from build123d import *

# Parameters (mm, degrees)
F1_DEPTH = 50


# Not quite as in the source:
# - ends of sketch curves that miss each other by under 0.0002 mm in the source are joined


with BuildPart() as f1:
    # F0 (on Front) → F1 (new body, symmetric)
    with BuildSketch(Plane.XZ):
        with BuildLine():
            Line((53.992555, -15.220268), (57.083133, -14.095389))
            ThreePointArc((57.083133, -14.095389), (62.9018568836, -10.252747544), (66.3544503107, -4.1944440905))
            ThreePointArc((66.3544503107, -4.1944440905), (66.1141142416, -2.8747683688), (64.914288, -2.275))
            Line((64.914288, -2.275), (60.670593, -2.275))
            ThreePointArc((60.670593, -2.275), (59.8472095147, -2.5211899521), (59.2941043505, -3.1789471518))
            ThreePointArc((59.2941043505, -3.1789471518), (56.9827494729, -6.2209259886), (53.52425904, -7.8441451998))
            ThreePointArc((53.52425904, -7.8441451998), (52.6431740995, -8.0626756758), (51.7855370008, -8.3602070021))
            ThreePointArc((51.7855370008, -8.3602070021), (39.452831, 0), (51.7855371982, 8.3602074972))
            ThreePointArc((51.7855371982, 8.3602074972), (52.6431743712, 8.0626765952), (53.524259133, 7.844145664))
            ThreePointArc((53.524259133, 7.844145664), (56.9827494729, 6.2209259886), (59.2941043849, 3.1789471667))
            ThreePointArc((59.2941043849, 3.1789471667), (59.8472095147, 2.5211899521), (60.670593, 2.275))
            Line((60.670593, 2.275), (64.914288, 2.275))
            ThreePointArc((64.914288, 2.275), (66.1141145297, 2.8747687527), (66.3544497778, 4.1944449353))
            ThreePointArc((66.3544497778, 4.1944449353), (62.9018565554, 10.2527478944), (57.0831331177, 14.0953893235))
            Line((57.0831331177, 14.0953893235), (53.992555, 15.220268))
            ThreePointArc((53.992555, 15.220268), (52.3736165632, 15.715360306), (50.7118440801, 16.0387645685))
            Line((50.7118440801, 16.0387645685), (40.585713, 17.465))
            Line((40.585713, 17.465), (35.885713, 17.465))
            ThreePointArc((35.885713, 17.465), (35.6735809656, 17.5528679656), (35.585713, 17.765))
            Line((35.585713, 17.765), (35.585713, 18.7))
            ThreePointArc((35.585713, 18.7), (35.4978450344, 18.9121320344), (35.285713, 19))
            Line((35.285713, 19), (18.585713, 19))
            Line((18.585713, 19), (12.836393, 18.04178))
            ThreePointArc((12.836393, 18.04178), (12.656806899, 17.9397743434), (12.585713, 17.745862))
            Line((12.585713, 17.745862), (12.585713, 6.875))
            ThreePointArc((12.585713, 6.875), (12.6735809656, 6.6628679656), (12.885713, 6.575))
            Line((12.885713, 6.575), (18.285713, 6.575))
            ThreePointArc((18.285713, 6.575), (18.4978450344, 6.6628679656), (18.585713, 6.875))
            Line((18.585713, 6.875), (18.585713, 12.7))
            ThreePointArc((18.585713, 12.7), (18.6735809656, 12.9121320344), (18.885713, 13))
            Line((18.885713, 13), (26.285713, 13))
            ThreePointArc((26.285713, 13), (26.4978450344, 12.9121320344), (26.585713, 12.7))
            Line((26.585713, 12.7), (26.585713, 10.3))
            ThreePointArc((26.585713, 10.3), (26.6735809656, 10.0878679656), (26.885713, 10))
            Line((26.885713, 10), (32.285713, 10))
            ThreePointArc((32.285713, 10), (32.4978450344, 9.9121320344), (32.585713, 9.7))
            Line((32.585713, 9.7), (32.585713, -9.7))
            ThreePointArc((32.585713, -9.7), (32.4978450344, -9.9121320344), (32.285713, -10))
            Line((32.285713, -10), (26.885713, -10))
            ThreePointArc((26.885713, -10), (26.6735809656, -10.0878679656), (26.585713, -10.3))
            Line((26.585713, -10.3), (26.585713, -12.7))
            ThreePointArc((26.585713, -12.7), (26.4978450344, -12.9121320344), (26.285713, -13))
            Line((26.285713, -13), (18.885713, -13))
            ThreePointArc((18.885713, -13), (18.6735809656, -12.9121320344), (18.585713, -12.7))
            Line((18.585713, -12.7), (18.585713, -6.875))
            ThreePointArc((18.585713, -6.875), (18.4978450344, -6.6628679656), (18.285713, -6.575))
            Line((18.285713, -6.575), (12.885713, -6.575))
            ThreePointArc((12.885713, -6.575), (12.6735809656, -6.6628679656), (12.585713, -6.875))
            Line((12.585713, -6.875), (12.585713, -17.745862))
            ThreePointArc((12.585713, -17.745862), (12.656806899, -17.9397743434), (12.8363929795, -18.0417801231))
            Line((12.8363929795, -18.0417801231), (18.585713, -19))
            Line((18.585713, -19), (35.285713, -19))
            ThreePointArc((35.285713, -19), (35.4978450344, -18.9121320344), (35.585713, -18.7))
            Line((35.585713, -18.7), (35.585713, -17.765))
            ThreePointArc((35.585713, -17.765), (35.6735809656, -17.5528679656), (35.885713, -17.465))
            Line((35.885713, -17.465), (40.585713, -17.465))
            Line((40.585713, -17.465), (50.711844, -16.038764))
            ThreePointArc((50.711844, -16.038764), (52.3736165632, -15.715360306), (53.992555, -15.220268))
        make_face()
    extrude(amount=F1_DEPTH, both=True)


solid = f1.part
Read the model definition and answer for the solid it produces. Units are mm, in the model's axes. A direction names the side the tool comes from. Round coordinates to 2 decimals unless told otherwise and drop trailing zeros. Write each loop counter-clockwise with the first axis right and the second up, starting at its lowest first coordinate (ties: lowest second). Pieces come first, ordered by that corner, then holes.
Q1. The mould has two halves that part along Z. Classify faces 1 (the face through (38, -1, -17.465)), 2 (the face through (45.72, -0.7, 16.74)), 3 (the face through (32.586, -1, 0)): released by +Z, released by -Z, zero draft, split by the parting line, or undercut.
Values:
face 1: released by -Z
face 2: released by +Z
face 3: undercut
Q2. Flat-ended cylindrical pins translate along their axes: P1, Ø0.5, axis at y = -6.5, z = 18, coming from the +X side; P2, Ø6, axis at y = -17, z = 3.5, coming from the -X side; P3, Ø1.5, axis at x = 45, y = 13.5, coming from the -Z side. Find the tip coordinate at first contact, or state that the pin passes through.
Values:
P1: stops at x = 35.59
P2: stops at x = 32.59
P3: stops at z = -16.95
Q3. Find section B-B on z = 0. Determine the outline of the cut face in (x, y), and give its area (3 significant figures).
Values:
outline: (32.59, -50) - (39.45, -50) - (39.45, 50) - (32.59, 50) - close
area: 687 mm2
Q4. Find section C-C on x = 63.5. Determine the outline of the cut face in (y, z) (3 decimals).
Values:
outline: (-50, -9.574) - (50, -9.574) - (50, -2.275) - (-50, -2.275) - close; (-50, 2.275) - (50, 2.275) - (50, 9.574) - (-50, 9.574) - close
Q5. Straight lines are drawn through the part: line 1 (Z direction, x = 24, y = -21.5); line 2 (X direction, y = -15, z = 0); line 3 (Z direction, x = 61.5, y = 22) (3 decimals). For each, find the intervals that lie inside material, in ascending order.
Values:
line 1: z = -19 to -13, 13 to 19
line 2: x = 32.59 to 39.45
line 3: z = -11.569 to -2.275, 2.275 to 11.569
Q6. Find section A-A on x = 28.5. Determine the outline of the cut face in (y, z), and give its area (3 significant figures).
Values:
outline: (-50, -19) - (50, -19) - (50, -10) - (-50, -10) - close; (-50, 10) - (50, 10) - (50, 19) - (-50, 19) - close
area: 1,800 mm2
Q7. A tool of negligible diameter and unlimited length cuts with its end or side. For faces 4 (the face through (16, -1, 6.575)), 5 (the face through (63, -1, -2.275)), 6 (the face through (30, -1, -10)), from which of +Z, -Z, +X, -X, +Y, -Y can it reach the whole face along a straight path? Write none if from no direction.
Values:
face 4: -X, +Y, -Y
face 5: +X, +Y, -Y
face 6: +Y, -Y
